Can you work these out from the model? Positions are in its coordinate system, mm. Coordinates: 2 decimals unless noted, no trailing zeros. Order: outer loops, then holes, each group sorted by start corner. A loop starts at its lowest first (then second) coordinate and runs counter-clockwise, first axis right, second up. Notation, with made-up numbers: M 68.25,39.5 L 80.25,39.5 A35 ccw 80.25,78.5 Z; hole C -11.5,-32 d9. An arc over 180 degrees is marked long. Answer as a JSON object with one key per item and string values.
from build123d import *

# Parameters (mm, degrees)
F0_R     = 11.43
F0_R_2   = 14.2875
F1_DEPTH = 25.4


with BuildPart() as f1:
    # F0 (on Top) → F1 (new body)
    with BuildSketch(Plane.XY):
        with BuildLine():
            ThreePointArc((-223.765199, 69.128216), (-207.381781, 65.700199), (-200.028299, 50.663778))
            ThreePointArc((-200.028299, 50.663778), (-207.723462, 35.367694), (-224.592098, 32.429181))
            Line((-224.592098, 32.429181), (-62.436875, -16.603506))
            ThreePointArc((-62.436875, -16.603506), (-73.880053, 24.794703), (-31.581428, 17.33921))
            ThreePointArc((-31.581428, 17.33921), (-32.128705, 48.14231), (-11.712275, 71.213935))
            ThreePointArc((-11.712275, 71.213935), (-47.089563, 84.80489), (-29.584343, 118.417891))
            Line((-29.584343, 118.417891), (-223.765199, 69.128216))
        make_face()
        with BuildLine():
            ThreePointArc((-224.592098, 32.429181), (-207.723462, 35.367694), (-200.028299, 50.663778))
            ThreePointArc((-200.028299, 50.663778), (-207.381781, 65.700199), (-223.765199, 69.128216))
            ThreePointArc((-223.765199, 69.128216), (-238.123465, 51.092902), (-224.592098, 32.429181))
        make_face()
        with Locations((-219.078299, 50.663778)):
            Circle(F0_R, mode=Mode.SUBTRACT)
        with BuildLine():
            ThreePointArc((2.064857, 93.79864), (-7.739786, 113.847202), (-29.584343, 118.417891))
            ThreePointArc((-29.584343, 118.417891), (-47.089563, 84.80489), (-11.712275, 71.213935))
            ThreePointArc((-11.712275, 71.213935), (-1.651268, 80.571034), (2.064857, 93.79864))
        make_face()
        with Locations((-23.335143, 93.79864)):
            Circle(F0_R_2, mode=Mode.SUBTRACT)
        with BuildLine():
            ThreePointArc((-31.581428, 17.33921), (-73.880053, 24.794703), (-62.436875, -16.603506))
            ThreePointArc((-62.436875, -16.603506), (-39.945361, -12.685489), (-29.685143, 7.70929))
            ThreePointArc((-29.685143, 7.70929), (-30.163723, 12.616714), (-31.581428, 17.33921))
        make_face()
        with Locations((-55.085143, 7.70929)):
            Circle(F0_R_2, mode=Mode.SUBTRACT)
    extrude(amount=F1_DEPTH)


solid = f1.part
Item 1: If we mould it in two halves opening along Y, with no side actions, what happens to faces 1 (the flat face through (-93, 52, 25.4)), 2 (the cylindrical face through (-238.113, 51.439, 12.522)), 3 (the cylindrical face through (-15.654, 105.846, 12.522))? For each: pulls with the +Y half, pulls with the -Y half, needs draft (parallel to the pull), parting line crosses it, or undercut.
Answers follow:
{"face 1": "needs draft", "face 2": "parting line crosses it", "face 3": "undercut"}
Item 2: I want a section at B-B, the plane z = 3.25. Give the number of separate pieces and of enclosed holes in the cut face, plus the area to 3 significant figures.
Answers follow:
{"separate pieces": "1", "enclosed holes": "3", "area": "17,400 mm^2"}
Item 3: I'm going to push flat-ended pins straight in: pin 1 (3 mm diameter, centred on y = 58.5, z = 9, fed in from +X); pin 2 (10 mm diameter, centred on x = -129, z = 8, fed in from -Y); pin 3 (12 mm diameter, centred on x = -30, z = 8.5, fed in from -Y). Where does each tip first touch, or does it pass through?
Answers follow:
{"pin 1": "stops at x = -25.43", "pin 2": "stops at y = 2.01", "pin 3": "stops at y = -9.05"}
Item 4: I want a section at D-D, the plane x = -162.5. Write out the boundary of the cut face in (y, z).
Answers follow:
{"outline": "M 13.65,0 L 84.68,0 L 84.68,25.4 L 13.65,25.4 Z"}
Item 5: Please list where these lines run through material, in increasing order: line 1 (X direction, y = 45.5, z = 24.25); line 2 (Y direction, x = -67.5, z = 22.25); line 3 (Y direction, x = -39, z = 21.25).
Answers follow:
{"line 1": "x = -237.42 to -229.28, -208.88 to -33.01", "line 2": "y = -15.07 to 0.64, 14.78 to 108.79", "line 3": "y = -11.95 to 116.03"}
Item 6: I want a section at A-A, the plane y = 14. Write out the boundary of the cut face in (x, z).
Answers follow:
{"outline": "M -163.65,0 L -67.91,0 L -67.91,25.4 L -163.65,25.4 Z; M -42.26,0 L -30.48,0 L -30.48,25.4 L -42.26,25.4 Z"}
Item 7: I want a section at C-C, the plane x = -211. Write out the boundary of the cut face in (y, z).
Answers follow:
{"outline": "M 28.32,0 L 42.58,0 L 42.58,25.4 L 28.32,25.4 Z; M 58.75,0 L 72.37,0 L 72.37,25.4 L 58.75,25.4 Z"}
